Geometry check sheet. Reference: drawing and pictorial views, mm from the part's lowest x, y, z. A direction names the side the tool comes from. Coordinates: 2 decimals unless noted, no trailing zeros. Write each loop counter-clockwise with the first axis right and the second up, starting at its lowest first coordinate (ties: lowest second). Pieces come first, ordered by that corner, then holes. Notation, with made-up numbers: (32, -24) - (46, -24) arc R20 ccw to (46, -14) - close; hole circle Ø8 at (70.25, 40). An arc over 180 degrees is marked (long way). Answer as a JSON object with one key per item and string values. Group by question number.
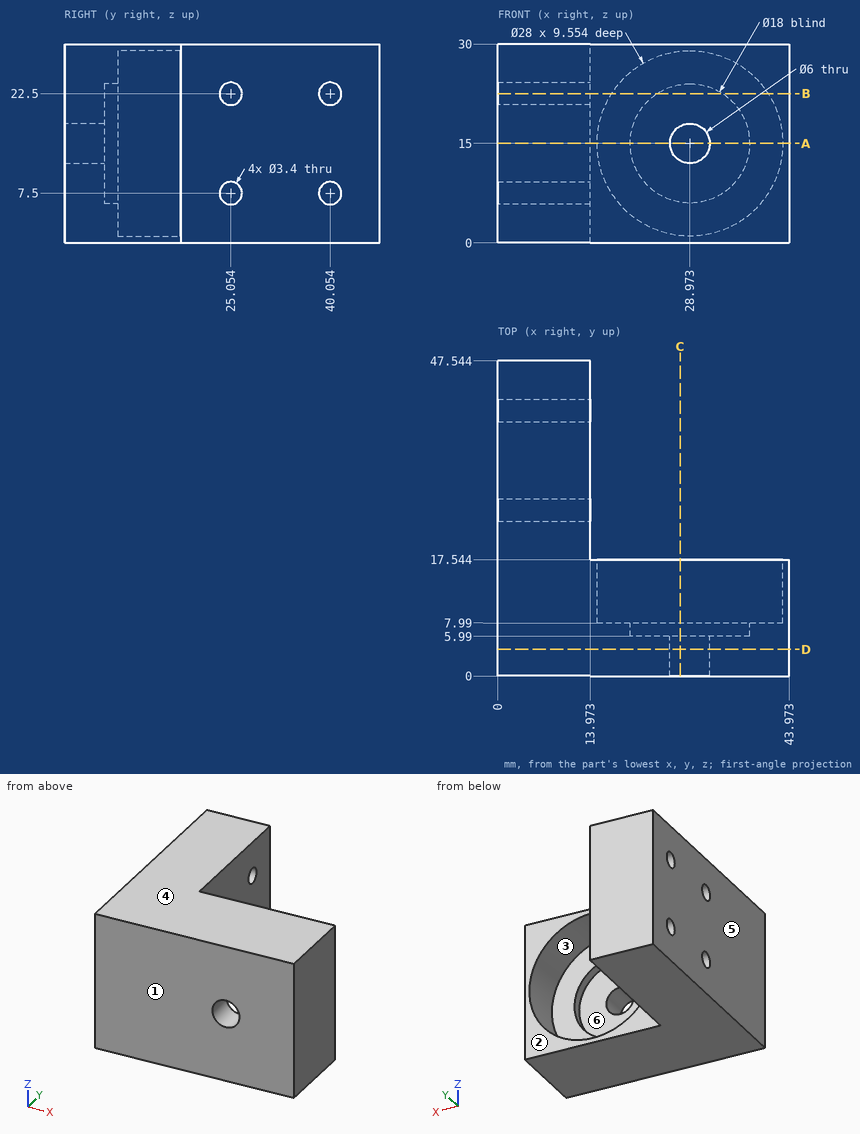
(1) Draft check along Z on the marked faces 4, 5 and 6. Enter one of: +Z half, -Z half, draft (parallel to the pull), parting line (faces both ways), or undercut.
(2) Section check C-C (x = 27.5). Record the cut outline in (y, z).
(3) Section check B-B (z = 22.5). Record the cut outline in (x, y), and give its area (3 significant figures).
(4) Material ranges on L1, parallel to Z at x = 3, y = 25; L2, parallel to Y at x = 10, z = 7.5; L3, parallel to Z at x = 28.5, y = 13.5, recorded low to high. Write a range as [from, to].
(5) Gauge pin test, flat ends, axial feed: pin 1 (14 mm diameter, centred on x = 33.5, z = 11.5, fed in from +Y); pin 2 (3 mm diameter, centred on y = 25.054, z = 22.5, fed in from -X); pin 3 (9 mm diameter, centred on x = 31.5, z = 17.5, fed in from +Y); pin 4 (4 mm diameter, centred on y = 20, z = 20.5, fed in from +X). Record the tip position at first contact, or that the pin passes through.
(6) Set-up check for the marked faces 1, 2 and 3: record each of +Z, -Z, +X, -X, +Y, -Y from which the full face is reachable in a straight line by a thin tool's end or side.
(7) Section check A-A (z = 15). Record the cut outline in (x, y), and give its area (3 significant figures).
(8) Section check D-D (y = 4). Record the cut outline in (x, z), and give its area (3 significant figures).
Conclusion:
{
 "1": {"face 4": "+Z half", "face 5": "draft", "face 6": "undercut"},
 "2": {"outline": "(0, 0) - (17.54, 0) - (17.54, 1.08) - (7.99, 1.08) - (7.99, 6.12) - (5.99, 6.12) - (5.99, 12.39) - (0, 12.39) - close; (0, 17.61) - (5.99, 17.61) - (5.99, 23.88) - (7.99, 23.88) - (7.99, 28.92) - (17.54, 28.92) - (17.54, 30) - (0, 30) - close"},
 "3": {"outline": "(0, 0) - (43.97, 0) - (43.97, 17.54) - (40.79, 17.54) - (40.79, 7.99) - (33.95, 7.99) - (33.95, 5.99) - (24, 5.99) - (24, 7.99) - (17.15, 7.99) - (17.15, 17.54) - (13.97, 17.54) - (13.97, 23.35) - (0, 23.35) - close; (0, 26.75) - (13.97, 26.75) - (13.97, 38.35) - (0, 38.35) - close; (0, 41.75) - (13.97, 41.75) - (13.97, 47.54) - (0, 47.54) - close", "area": "850 mm^2"},
 "4": {"L1": "z = [0, 5.8], [9.2, 20.8], [24.2, 30]", "L2": "y = [0, 23.35], [26.75, 38.35], [41.75, 47.54]", "L3": "z = [0, 1.01], [28.99, 30]"},
 "5": {"pin 1": "stops at y = 7.99", "pin 2": "passes through", "pin 3": "stops at y = 5.99", "pin 4": "stops at x = 13.97"},
 "6": {"face 1": "+Z, -Z, +X, -X, -Y", "face 2": "+Z, -Z, +X, +Y", "face 3": "+Y"},
 "7": {"outline": "(0, 0) - (25.97, 0) - (25.97, 5.99) - (19.97, 5.99) - (19.97, 7.99) - (14.97, 7.99) - (14.97, 17.54) - (13.97, 17.54) - (13.97, 47.54) - (0, 47.54) - close; (31.97, 0) - (43.97, 0) - (43.97, 17.54) - (42.97, 17.54) - (42.97, 7.99) - (37.97, 7.99) - (37.97, 5.99) - (31.97, 5.99) - close", "area": "851 mm^2"},
 "8": {"outline": "(0, 0) - (43.97, 0) - (43.97, 30) - (0, 30) - close; hole circle Ø6 at (28.97, 15)", "area": "1,290 mm^2"}
}
